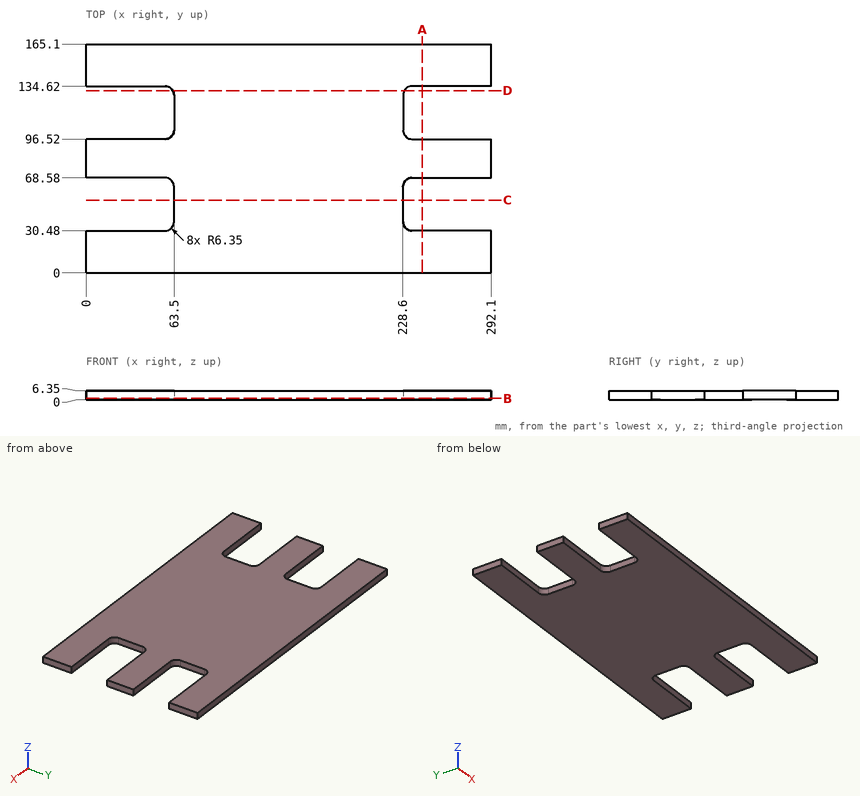
Print and shaded views of the part. All mm, measured from the part's lowest x, y and z. Coordinates: 2 decimals unless noted, no trailing zeros. Order: outer loops, then holes, each group sorted by start corner. A loop starts at its lowest first (then second) coordinate and runs counter-clockwise, first axis right, second up. Notation, with made-up numbers: (31, -28.5) -> (85, -28.5) arc R29 ccw to (85, -6.5) -> close; hole circle Ø11 at (-25.75, 78.5). An arc over 180 degrees is marked (long way). Use one line per item in the form item = value. Start each with the question number.
1) Drill centre lines: L1, parallel to Y at x = 55, z = 0.75; L2, parallel to X at y = 46.5, z = 6.25; L3, parallel to X at y = 33.5, z = 1.75. Where is each one in solid material? Low to high. Write a range as [from, to].
2) Band-saw the part on C-C on y = 52.5. Give the cut face in (x, z).
3) Drop flat-ended pins along their axis: pin 1 (3 mm diameter, centred on y = 47, z = 4, fed in from -X); pin 2 (3 mm diameter, centred on y = 112.5, z = 2.5, fed in from +X). Give the stop position or say it passes through.
4) Band-saw the part on A-A on x = 242.5. Give the cut face in (y, z), then the cut area to 3 significant figures.
5) Band-saw the part on D-D on y = 131.5. Give the cut face in (x, z).
6) Band-saw the part on B-B on z = 1. Give the cut face in (x, y), then the cut area to 3 significant figures.
Entries:
q1.L1 = [0, 30.48], [68.58, 96.52], [134.62, 165.1]
q1.L2 = [63.5, 228.6]
q1.L3 = [62.56, 229.54]
q2.outline = (63.5, 0) -> (228.6, 0) -> (228.6, 6.35) -> (63.5, 6.35) -> close
q3.pin_1 = 63.5
q3.pin_2 = 228.6
q4.outline = (0, 0) -> (30.48, 0) -> (30.48, 6.35) -> (0, 6.35) -> close; (68.58, 0) -> (96.52, 0) -> (96.52, 6.35) -> (68.58, 6.35) -> close; (134.62, 0) -> (165.1, 0) -> (165.1, 6.35) -> (134.62, 6.35) -> close
q4.area = 565 mm2
q5.outline = (62.62, 0) -> (229.48, 0) -> (229.48, 6.35) -> (62.62, 6.35) -> close
q6.outline = (0, 0) -> (292.1, 0) -> (292.1, 30.48) -> (234.95, 30.48) arc R6.35 cw to (228.6, 36.83) -> (228.6, 62.23) arc R6.35 cw to (234.95, 68.58) -> (292.1, 68.58) -> (292.1, 96.52) -> (234.95, 96.52) arc R6.35 cw to (228.6, 102.87) -> (228.6, 128.27) arc R6.35 cw to (234.95, 134.62) -> (292.1, 134.62) -> (292.1, 165.1) -> (0, 165.1) -> (0, 134.62) -> (57.15, 134.62) arc R6.35 cw to (63.5, 128.27) -> (63.5, 102.87) arc R6.35 cw to (57.15, 96.52) -> (0, 96.52) -> (0, 68.58) -> (57.15, 68.58) arc R6.35 cw to (63.5, 62.23) -> (63.5, 36.83) arc R6.35 cw to (57.15, 30.48) -> (0, 30.48) -> close
q6.area = 38,600 mm2
